from build123d import *

# Parameters (mm, degrees)
F1_R      = 12.5
F4_DEPTH  = 0.5
F5_R      = 4
F6_DEPTH  = 0.5
F3_R      = 3
F2_R      = 2.7
F7_R      = 3
F9_DEPTH  = 25
F14_DEPTH = 0.5


with BuildPart() as f4:
    # F1 (on Front) → F4 (new body)
    with BuildSketch(Plane.XZ):
        Circle(F1_R)
    extrude(amount=F4_DEPTH)

    # F5 (on face) → F6 (join)
    with BuildSketch(Plane.XZ.offset(0.5)):
        Circle(F5_R)
    extrude(amount=F6_DEPTH)

    # F3 (on Front) → F8 section 0
    with BuildSketch(Plane.XZ):
        Circle(F3_R)
    # F2 (on offset) → F8 section 1
    with BuildSketch(Plane.XZ.offset(1.5)):
        Circle(F2_R)
    loft(mode=Mode.SUBTRACT)

    # F7 (on face) → F9 (cut)
    with BuildSketch(Plane.XZ.offset(1)):
        Circle(F7_R)
    extrude(amount=-F9_DEPTH, mode=Mode.SUBTRACT)


with BuildPart() as f10_1:
    # F10: copy of F4
    add(f4.part.moved(Location((35, 0, 0))))


with BuildPart() as f11_1:
    # F11: copy of F4
    add(f4.part.moved(Location((105, 0, 0))))


with BuildPart() as f12_1:
    # F12: copy of F4
    add(f4.part.moved(Location((70, 0, 0))))


with BuildPart() as f4_1:
    add(f4.part)

    add(f10_1.part)  # F14 merges F10_1

    add(f11_1.part)  # F14 merges F11_1

    add(f12_1.part)  # F14 merges F12_1
    # F13 (on Front) → F14 (join)
    with BuildSketch(Plane.XZ):
        with BuildLine():
            ThreePointArc((27.0678855609, 9.6608260788), (17.5, 6.5713974561), (7.9321144391, 9.6608260788))
            Line((7.9321144391, 9.6608260788), (7.9321144391, -9.6608260788))
            ThreePointArc((7.9321144391, -9.6608260788), (17.5, -6.5713974561), (27.0678855609, -9.6608260788))
            Line((27.0678855609, -9.6608260788), (27.0678855609, 9.6608260788))
        make_face()
        with BuildLine():
            ThreePointArc((62.0678855609, 9.6608260788), (52.5, 6.5713974561), (42.9321144391, 9.6608260788))
            Line((42.9321144391, 9.6608260788), (42.9321144391, -9.6608260788))
            ThreePointArc((42.9321144391, -9.6608260788), (52.5, -6.5713974561), (62.0678855609, -9.6608260788))
            Line((62.0678855609, -9.6608260788), (62.0678855609, 9.6608260788))
        make_face()
        with BuildLine():
            ThreePointArc((97.0678855609, 9.6608260788), (87.5, 6.5713974561), (77.9321144391, 9.6608260788))
            Line((77.9321144391, 9.6608260788), (77.9321144391, -9.6608260788))
            ThreePointArc((77.9321144391, -9.6608260788), (87.5, -6.5713974561), (97.0678855609, -9.6608260788))
            Line((97.0678855609, -9.6608260788), (97.0678855609, 9.6608260788))
        make_face()
    extrude(amount=F14_DEPTH)


solid = f4_1.part
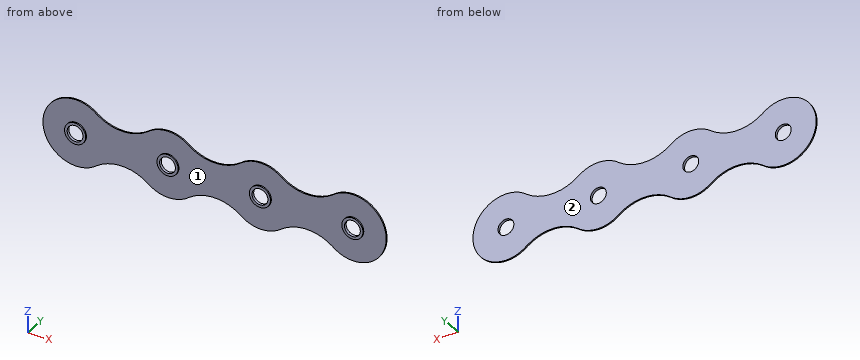
CAD build for the part. Positions are in the model's coordinates, mm. Face numbers are marked on the shaded views. Give positions to 0.01 mm unless a question says otherwise; leave off trailing zeros. Order: outer loops, then holes, each group sorted by start corner. A loop starts at its lowest first (then second) coordinate and runs counter-clockwise, first axis right, second up. Notation, with made-up numbers: (58.5, 75.5) -> (117.5, 75.5) arc R21 ccw to (117.5, 83.5) -> close; hole circle Ø9 at (86, 82.5). An arc over 180 degrees is marked (long way). Return JSON: item names as keys, results as strings.
Q1. Flat gauge pins, fed straight in: pin 1 (8 mm diameter, centred on x = 0, z = 0, fed in from +Y); pin 2 (3 mm diameter, centred on x = 62, z = 0, fed in from -Y). Where does each tip first touch, or does it go through?
Working result:
{"pin 1": "y = 0", "pin 2": "y = -0.5"}
Q2. Saw through at B-B (x = 70). Write the cut outline in (y, z), then the cut area to 3 significant figures.
Working result:
{"outline": "(-1, -4) -> (-0.5, -4) -> (-0.5, -12.5) -> (0, -12.5) -> (0, -3) -> (-1, -3) -> close; (-1, 3) -> (0, 3) -> (0, 12.5) -> (-0.5, 12.5) -> (-0.5, 4) -> (-1, 4) -> close", "area": "10.5 mm²"}
Q3. Mould opens along X. For the marked faces 1 and 2 say: pulls with the +X half, pulls with the -X half, needs draft (parallel to the pull), parting line crosses it, or undercut.
Working result:
{"face 1": "undercut", "face 2": "needs draft"}
Q4. Saw through at A-A (y = -0.7). Write the cut outline in (x, z).
Working result:
{"outline": "circle Ø8 at (0, 0); circle Ø8 at (35, 0); circle Ø8 at (70, 0); circle Ø8 at (105, 0); hole circle Ø6 at (0, 0); hole circle Ø6 at (35, 0); hole circle Ø6 at (70, 0); hole circle Ø6 at (105, 0)"}
Q5. Saw through at C-C (z = 8.5). Write the cut outline in (x, y), then the cut area to 3 significant figures.
Working result:
{"outline": "(-9.17, -0.5) -> (9.79, -0.5) -> (9.79, 0) -> (-9.17, 0) -> close; (25.21, -0.5) -> (44.79, -0.5) -> (44.79, 0) -> (25.21, 0) -> close; (60.21, -0.5) -> (79.79, -0.5) -> (79.79, 0) -> (60.21, 0) -> close; (95.21, -0.5) -> (114.17, -0.5) -> (114.17, 0) -> (95.21, 0) -> close", "area": "38.5 mm²"}
Q6. Drill centre lines: line 1 (X direction, y = -0.4, z = -11); line 2 (Z direction, x = 0, y = -0.55); line 3 (X direction, y = -0.35, z = 2). Where is each one in solid material? Low to high.
Working result:
{"line 1": "-5.94 to 5.94, 29.06 to 40.94, 64.06 to 75.94, 99.06 to 110.94", "line 2": "-4 to -3, 3 to 4", "line 3": "-12.34 to -2.24, 2.24 to 32.76, 37.24 to 67.76, 72.24 to 102.76, 107.24 to 117.34"}
Q7. Saw through at D-D (z = 0). Count the separate pieces of the cut face and the enclosed holes in it, then the cut area to 3 significant figures.
Working result:
{"separate pieces": "5", "enclosed holes": "0", "area": "57.0 mm²"}
